Geometry: final body of the model. Coordinates: model frame, mm. A direction names the side the tool comes from. Give positions to 0.01 mm unless a question says otherwise; leave off trailing zeros. Loops run counter-clockwise (first coordinate to the right, second up) from the corner with the lowest first, then second, coordinate; pieces in that order, holes last. Notation, with made-up numbers: (21.5, 65) -> (35.5, 65) arc R29 ccw to (35.5, 96) -> close; hole circle Ø9 at (54.5, 38.5). An arc over 180 degrees is marked (long way). Answer in a Markdown table with one row per item. Add a question column.
1) Section query B-B (x = -277). Return the cut outline in (y, z).
2) Section query A-A (x = 975). Return the cut outline in (y, z), plus the area to 3 significant figures.
3) First-contact query: P1, Ø4, axis at y = 52.5, z = 77, coming from the -X side; P2, Ø6, axis at x = 910.5, y = -2, coming from the +Z side; P3, Ø4, axis at x = 770, z = 12.5, coming from the -Y side; P4, Ø8, axis at x = 818, y = 0.5, coming from the +Z side. Flat tips, straight axial feed; report the tip coordinate or a pass-through.
4) Section query C-C (x = 52). Return the cut outline in (y, z).
5) Access query for faces 4 (the cylindrical face through (-842.325, 209.887, -46.608)), 5 (the cylindrical face through (-779.3, -202.37, 129.02)), 6 (the cylindrical face through (656.27, 79.845, 41.53)), 7 (the flat face through (830, -90, -197)). Directions: +Z, -Z, +X, -X, +Y, -Y. A direction counts if a zero-diameter tool reaches every point of the face in a straight line with its end or side. Return the directions, or none.
6) Line query: line 1 (X direction, y = 62, z = 127); line 2 (Z direction, x = 451.5, y = -3); line 3 (X direction, y = -80, z = -73.5). Output: solid intervals per line, ascending. Write a range as from..to.
7) Draft query along Y for faces 1 (the flat face through (855, -3, -3)), 2 (the flat face through (-830, -90, 197)), 3 (the cylindrical face through (842.675, 209.887, -46.608)). Return one class per face: +Y half, -Y half, draft (parallel to the pull), parting line (faces both ways), or undercut.
```python
from build123d import *

# Parameters (mm, degrees)
SKETCH2_R           = 15
BOSS_EXTRUDE1_DEPTH = 360


with BuildPart() as part:
    # Sketch1 → Revolve1 (revolve)
    with BuildSketch(Plane.XY, mode=Mode.PRIVATE) as revolve1_sk:
        with BuildLine():
            Line((-855, 0), (-855, 215))
            Line((-855, 215), (-830, 215))
            Line((-830, 215), (-830, 240))
            Line((-830, 240), (-730, 240))
            Line((-730, 240), (-705, 160))
            Line((-705, 160), (-705, 90))
            Line((-705, 90), (-606.156213382, 90))
            Line((-606.156213382, 90), (-606.156213382, 75))
            Line((-606.156213382, 75), (-129.903810568, 75))
            ThreePointArc((-129.903810568, 75), (0, 150), (129.903810568, 75))
            Line((129.903810568, 75), (606.156213382, 75))
            Line((606.156213382, 75), (606.156213382, 90))
            Line((606.156213382, 90), (705, 90))
            Line((705, 90), (705, 160))
            Line((705, 160), (730, 240))
            Line((730, 240), (830, 240))
            Line((830, 240), (830, 215))
            Line((830, 215), (855, 215))
            Line((855, 215), (855, 0))
            Line((855, 0), (-855, 0))
        make_face()
    revolve(revolve1_sk.sketch.rotate(Axis((-1250, 0, 0), (1, 0, 0)), 90), axis=Axis((-1250, 0, 0), (1, 0, 0)))

    # Sketch2 → Boss-Extrude1 (add)
    with BuildSketch(Plane.ZY.offset(855)):
        with Locations(Location((0, 150, 0), (0, 0, 180))):
            Circle(SKETCH2_R)
        with Locations(Location((106.066017178, 106.066017178, 0), (0, 0, 180))):
            Circle(SKETCH2_R)
        with Locations(Location((150, 0, 0), (0, 0, 180))):
            Circle(SKETCH2_R)
        with Locations(Location((106.066017178, -106.066017178, 0), (0, 0, 180))):
            Circle(SKETCH2_R)
        with Locations(Location((0, -150, 0), (0, 0, 180))):
            Circle(SKETCH2_R)
        with Locations(Location((-106.066017178, -106.066017178, 0), (0, 0, 180))):
            Circle(SKETCH2_R)
        with Locations(Location((-150, 0, 0), (0, 0, 180))):
            Circle(SKETCH2_R)
        with Locations(Location((-106.066017178, 106.066017178, 0), (0, 0, 180))):
            Circle(SKETCH2_R)
    boss_extrude1 = extrude(amount=BOSS_EXTRUDE1_DEPTH)

    # Mirror1: Boss-Extrude1 across plane
    add(boss_extrude1.mirror(Plane(origin=(0, 0, 0), x_dir=(0, 0, 1), z_dir=(1, 0, 0))))


solid = part.part
```
Evaluation:
| question | item | result |
|---|---|---|
| 1 | outline | circle Ø150 at (0, 0) |
| 2 | outline | circle Ø30 at (-150, 0); circle Ø30 at (-106.07, -106.07); circle Ø30 at (-106.07, 106.07); circle Ø30 at (0, -150); circle Ø30 at (0, 150); circle Ø30 at (106.07, -106.07); circle Ø30 at (106.07, 106.07); circle Ø30 at (150, 0) |
| 2 | area | 5,650 mm² |
| 3 | P1 | x = -855 |
| 3 | P2 | z = 165 |
| 3 | P3 | y = -239.77 |
| 3 | P4 | z = 240 |
| 4 | outline | circle Ø281.4 at (0, 0) |
| 5 | face 4 | -X |
| 5 | face 5 | +X, -X |
| 5 | face 6 | none |
| 5 | face 7 | +X |
| 6 | line 1 | -855..-705, -50.27..50.27, 705..855 |
| 6 | line 2 | -74.94..74.94 |
| 6 | line 3 | -855..-705, -103.43..103.43, 705..855 |
| 7 | face 1 | undercut |
| 7 | face 2 | draft |
| 7 | face 3 | parting line |
